```python
from build123d import *

# Parameters (mm, degrees)
F1_DEPTH = 2.5
F3_DEPTH = 5
F4_R     = 1


# Not quite as in the source:
# - a feature names something its author has since deleted; it is built from what else it names


with BuildPart() as f1:
    # F0 (on Front) → F1 (new body, symmetric)
    with BuildSketch(Plane.XZ):
        Polygon((-6.985, -1.9016251091), (-12.7, -1.9016251091), (-12.7, -27.3016251091), (12.7, -27.3016251091), (12.7, -1.9016251091), (6.985, -1.9016251091), (0, -14), align=None)
    extrude(amount=F1_DEPTH, both=True)

    # F2 (on face) → F3 (join)
    with BuildSketch(Plane(origin=(0, 0, -27.3016251091), x_dir=(1, 0, 0), z_dir=(0, 0, -1))):
        with BuildLine():
            ThreePointArc((-12.7, -10), (-11.2355339059, -13.5355339059), (-7.7, -15))
            Line((-7.7, -15), (7.7, -15))
            ThreePointArc((7.7, -15), (11.2355339059, -13.5355339059), (12.7, -10))
            Line((12.7, -10), (12.7, -2.5))
            Line((12.7, -2.5), (-12.7, -2.5))
            Line((-12.7, -2.5), (-12.7, -10))
        make_face()
        with BuildLine():
            Line((-5, -7.5), (5, -7.5))
            ThreePointArc((5, -7.5), (7.5, -10), (5, -12.5))
            Line((5, -12.5), (-5, -12.5))
            ThreePointArc((-5, -12.5), (-7.5, -10), (-5, -7.5))
        make_face(mode=Mode.SUBTRACT)
    extrude(amount=-F3_DEPTH)

    # F4
    f4_edges = [f1.edges().sort_by_distance(p)[0] for p in [
        (-12.7, -2.5, -14.601625),
        (-9.8425, -2.5, -1.901625),
        (-12.7, 0, -1.901625),
        (-9.8425, 2.5, -1.901625),
        (-12.7, 2.5, -12.101625),
        (-12.7, 6.25, -22.301625),
        (12.7, 2.5, -12.101625),
        (12.7, -2.5, -14.601625),
        (12.7, 0, -1.901625),
        (9.8425, 2.5, -1.901625),
        (9.8425, -2.5, -1.901625),
    ]]
    fillet(f4_edges, radius=F4_R)


solid = f1.part
```
Could you check a few things on this model? Use its own coordinates, in mm. A direction names the side the tool comes from. Coordinates: 2 decimals unless noted, no trailing zeros. Order: outer loops, then holes, each group sorted by start corner. A loop starts at its lowest first (then second) coordinate and runs counter-clockwise, first axis right, second up. Notation, with made-up numbers: M -6.5,-12.75 L 31.5,-12.75 A19 ccw 31.5,-6.75 Z; hole C 88.25,-9.5 d11. An arc over 180 degrees is marked long. Use one line per item in the form item = value. Start each with the question number.
1. On a 3-axis mill with a long thin cutter (end or side, diameter ignored), from which of +Z, -Z, +X, -X, +Y, -Y can I reach the whole of each face in a straight line? I mean faces 1 (the cylindrical face through (-7.5, 10.1, -24.8)), 2 (the cylindrical face through (12.415, 2.199, -12.959)), 3 (the cylindrical face through (-12.399, 2.215, -13.244)), 4 (the flat face through (0, 2.5, -15)). Say none if no direction works.
2. For pin 1 (5 mm diameter, centred on x = 8, y = 11, fed in from +Z); pin 2 (1.5 mm diameter, centred on x = 6.5, y = 3, fed in from +Z); pin 3 (10 mm diameter, centred on y = 13, z = -14.5, fed in from -X), each with a flat end and sliding along its axis, tell me the tip position at first contact or that it passes through.
3. Please list where these lines run through material, in increasing order: line 1 (Z direction, x = -0.75, y = 4.75); line 2 (Y direction, x = 11, z = -10); line 3 (X direction, y = 0.25, z = -8).
4. Suppose I cut it at B-B on x = 2.5. Write out the boundary of the cut face in (y, z).
5. Suppose I cut it at A-A on y = 9. Write out the boundary of the cut face in (x, z), then the cut area to 3 significant figures.
6. We'd pull the mould along X, two halves only. Please class faces 5 (the cylindrical face through (-9.09, -2.21, -2.2)), 6 (the flat face through (3.54, -0.04, -7.87)), 7 (the flat face through (12.7, 0, -21)): +X half, -X half, draft (parallel to the pull), parting line (faces both ways), or undercut.
Geometry says:
q1.face_1 = +Z, -Z
q1.face_2 = +Z, +X, +Y
q1.face_3 = +Z, -X, +Y
q1.face_4 = +Z, +X, -X, +Y
q2.pin_1 = -22.3
q2.pin_2 = -2.3
q2.pin_3 = through
q3.line_1 = -27.3 to -22.3
q3.line_2 = -2.5 to 2.5
q3.line_3 = -12.7 to -3.46, 3.46 to 12.7
q4.outline = M -2.5,-27.3 L 7.5,-27.3 L 7.5,-22.3 L 2.5,-22.3 L 2.5,-9.67 L -2.5,-9.67 Z; M 12.5,-27.3 L 15,-27.3 L 15,-23.3 A1 ccw 14,-22.3 L 12.5,-22.3 Z
q5.outline = M -12.7,-27.3 L -7.29,-27.3 L -7.29,-22.3 L -11.7,-22.3 A1 ccw -12.7,-23.3 Z; M 7.29,-27.3 L 12.7,-27.3 L 12.7,-23.3 A1 ccw 11.7,-22.3 L 7.29,-22.3 Z
q5.area = 53.7 mm^2
q6.face_5 = draft
q6.face_6 = undercut
q6.face_7 = +X half
